Read the model definition and answer for the solid it produces. Units are mm, in the model's axes. Face numbers are marked on the shaded views. Coordinates: 2 decimals unless noted, no trailing zeros. Write each loop counter-clockwise with the first axis right and the second up, starting at its lowest first coordinate (ties: lowest second). Pieces come first, ordered by that corner, then holes.
(1) Find the intervals of material crossed by probe 1 along X at (y, z) = (6.5, -0.25); probe 2 along X at (y, z) = (2.5, -2.25), in increasing order.
(2) Section C-C on y = 3.25 is taken. Write down the section's boundary in (x, z) (1 decimal), then the cut area to 3 significant figures.
(3) Section A-A on x = 0 is taken. Write down the section's boundary in (y, z).
(4) The mould has two halves that part along Z. Classify the marked faces 1, 2 and 3: +Z half, -Z half, draft (parallel to the pull), parting line (faces both ways), or undercut.
(5) Section D-D on z = 8.5 is taken. Write down the section's boundary in (x, y), then the cut area to 3 significant figures.
(6) Given pin 1 (1 mm diameter, centred on x = -3.5, z = -5.5, fed in from -Y); pin 2 (1 mm diameter, centred on y = 6, z = -7.5, fed in from +X); pin 3 (1 mm diameter, centred on x = -2, y = 4, fed in from +Z); pin 4 (8.5 mm diameter, centred on x = 0, z = 0, fed in from +Y), each flat-ended and moving along its own axis, determine where each tip first touches the part or whether it passes through.
(7) Section B-B on z = 0 is taken. Write down the section's boundary in (x, y).
from build123d import *

# Parameters (mm, degrees)
SKETCH_1_R          = 12.3063
EXTRUDE_1_DEPTH     = 1.524
SKETCH_2_R          = 11.1125
EXTRUDE_2_DEPTH     = 5.588
SKETCH_3_R          = 4.7625
CUT_EXTRUDE_1_DEPTH = 8.112


with BuildPart() as part:
    # 草圖1 → 填料-伸長1 (new body)
    with BuildSketch(Plane(origin=(0, 0, 0), x_dir=(1, 0, 0), z_dir=(0, 1, 0))):
        Circle(SKETCH_1_R)
    extrude(amount=EXTRUDE_1_DEPTH)

    # 草圖2 → 填料-伸長2 (add)
    with BuildSketch(Plane(origin=(0, 1.524, 0), x_dir=(1, 0, 0), z_dir=(0, 1, 0))):
        Circle(SKETCH_2_R)
    extrude(amount=EXTRUDE_2_DEPTH)

    # 草圖3 → 除料-伸長1 (cut, through all)
    with BuildSketch(Plane(origin=(0, 7.112, 0), x_dir=(1, 0, 0), z_dir=(0, 1, 0))):
        Circle(SKETCH_3_R)
    extrude(amount=-CUT_EXTRUDE_1_DEPTH, mode=Mode.SUBTRACT)


solid = part.part
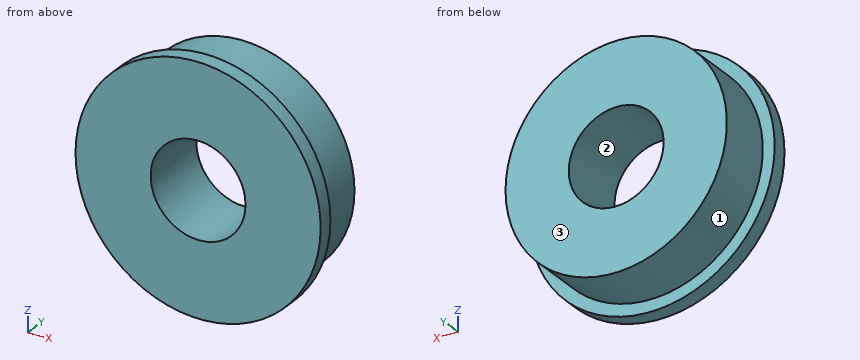
Response:
1. probe 1: x = -11.11 to -4.76, 4.76 to 11.11
1. probe 2: x = -10.88 to -4.2, 4.2 to 10.88
2. outline: circle Ø22.2 at (0, 0); hole circle Ø9.5 at (0, 0)
2. area: 317 mm2
3. outline: (0, -12.31) - (1.52, -12.31) - (1.52, -11.11) - (7.11, -11.11) - (7.11, -4.76) - (0, -4.76) - close; (0, 4.76) - (7.11, 4.76) - (7.11, 11.11) - (1.52, 11.11) - (1.52, 12.31) - (0, 12.31) - close
4. face 1: parting line
4. face 2: undercut
4. face 3: draft
5. outline: (-8.9, 0) - (8.9, 0) - (8.9, 1.52) - (7.16, 1.52) - (7.16, 7.11) - (-7.16, 7.11) - (-7.16, 1.52) - (-8.9, 1.52) - close
5. area: 107 mm2
6. pin 1: stops at y = 0
6. pin 2: stops at x = 8.63
6. pin 3: stops at z = 11.01
6. pin 4: passes through
7. outline: (-12.31, 0) - (-4.76, 0) - (-4.76, 7.11) - (-11.11, 7.11) - (-11.11, 1.52) - (-12.31, 1.52) - close; (4.76, 0) - (12.31, 0) - (12.31, 1.52) - (11.11, 1.52) - (11.11, 7.11) - (4.76, 7.11) - close
